Source: three-view drawing plus pictorial views. Frame: mm from the lowest corner of the part. Round coordinates to 2 decimals unless told otherwise and drop trailing zeros. Loops run counter-clockwise (first coordinate to the right, second up) from the corner with the lowest first, then second, coordinate; pieces in that order, holes last. Notation, with made-up numbers: (50, -6.75) -> (78, -6.75) arc R8 cw to (78, -1.75) -> close; hole circle Ø10 at (53.5, 30.5). An arc over 180 degrees is marked (long way). Put each result on its own line as item: value. Start each with the question number.
1. Material intervals for L1, parallel to Y at x = 45, z = 1.45 (3 decimals); L2, parallel to X at y = 46, z = 0.85; L3, parallel to Y at x = 4.5, z = 1.25, sorted ascending.
2. Cut plane B-B (y = 46.7). Return the cut outline in (x, z) (3 decimals), then the cut area to 3 significant figures.
3. Cut plane A-A (x = 45). Return the cut outline in (y, z) (3 decimals).
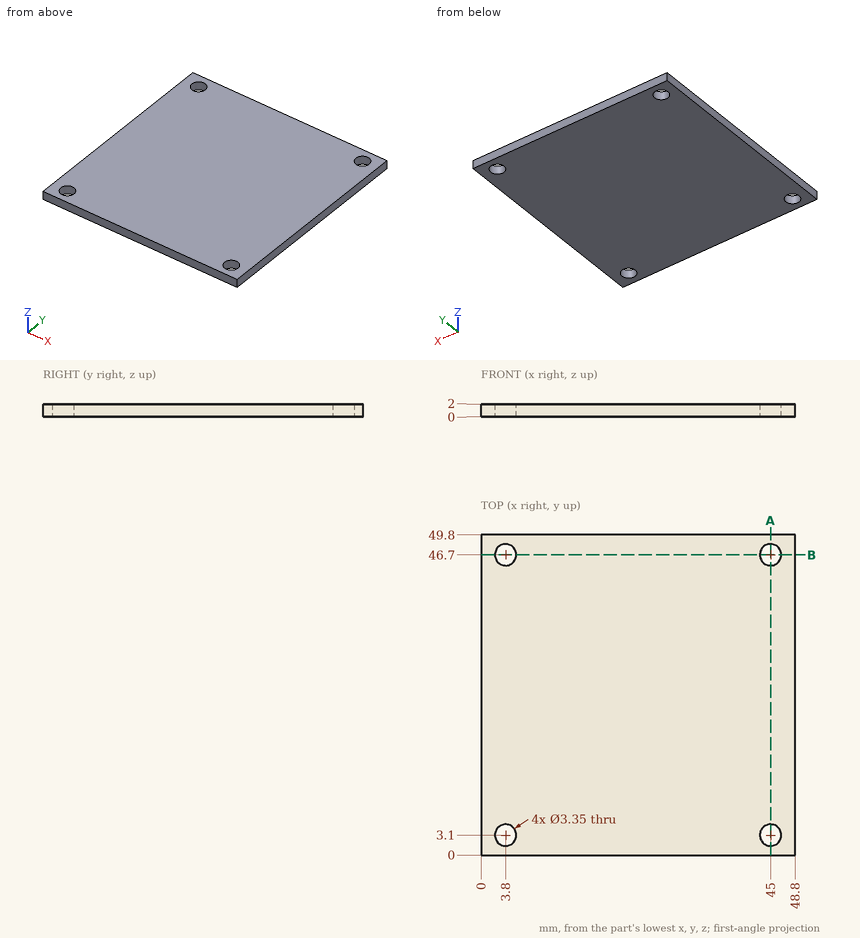
Solution:
1. L1: y = 0 to 1.425, 4.775 to 45.025, 48.375 to 49.8
1. L2: x = 0 to 2.28, 5.32 to 43.48, 46.52 to 48.8
1. L3: y = 0 to 1.58, 4.62 to 45.18, 48.22 to 49.8
2. outline: (0, 0) -> (2.125, 0) -> (2.125, 2) -> (0, 2) -> close; (5.475, 0) -> (43.325, 0) -> (43.325, 2) -> (5.475, 2) -> close; (46.675, 0) -> (48.8, 0) -> (48.8, 2) -> (46.675, 2) -> close
2. area: 84.2 mm^2
3. outline: (0, 0) -> (1.425, 0) -> (1.425, 2) -> (0, 2) -> close; (4.775, 0) -> (45.025, 0) -> (45.025, 2) -> (4.775, 2) -> close; (48.375, 0) -> (49.8, 0) -> (49.8, 2) -> (48.375, 2) -> close
